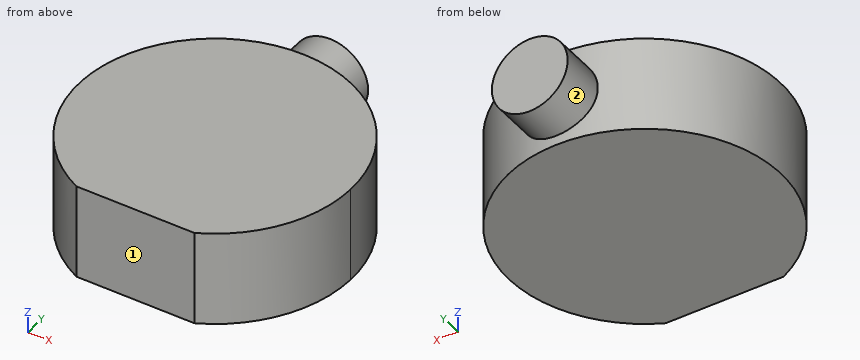
```python
from build123d import *

# Parameters (mm, degrees)
SKETCH_1_R          = 50
EXTRUDE_1_DEPTH     = 35
SKETCH_2_R          = 14
EXTRUDE_2_DEPTH     = 65
CUT_EXTRUDE_START   = -110
SKETCH_3_W          = 150
SKETCH_3_H          = 100
CUT_EXTRUDE_1_DEPTH = 64


with BuildPart() as part:
    # 草图1 → 凸台-拉伸1 (new body)
    with BuildSketch(Plane.XY):
        Circle(SKETCH_1_R)
    extrude(amount=EXTRUDE_1_DEPTH)

    # 草图2 → 凸台-拉伸2 (add)
    with BuildSketch(Plane(origin=(0, 0, 0), x_dir=(1, 0, 0), z_dir=(0, 1, 0))):
        with Locations((0, -17.5)):
            Circle(SKETCH_2_R)
    extrude(amount=EXTRUDE_2_DEPTH)

    # 草图3 → 切除-拉伸1 (cut)
    with BuildSketch(Plane(origin=(0, 65, 0), x_dir=(1, 0, 0), z_dir=(0, 1, 0)).offset(CUT_EXTRUDE_START)):
        Rectangle(SKETCH_3_W, SKETCH_3_H)
    extrude(amount=-CUT_EXTRUDE_1_DEPTH, mode=Mode.SUBTRACT)


solid = part.part
```
The listing builds one solid part. Answer for the finished solid, in the listing's coordinates (mm). Face numbers are marked on the shaded views. A direction names the side the tool comes from. Coordinates: 2 decimals unless noted, no trailing zeros. Write each loop counter-clockwise with the first axis right and the second up, starting at its lowest first coordinate (ties: lowest second). Pieces come first, ordered by that corner, then holes. Notation, with made-up numbers: (60.25, 33) - (110.25, 33) arc R26 ccw to (110.25, 70) - close; hole circle Ø10 at (-0.75, 67.5). An arc over 180 degrees is marked (long way). One line per item, written item: value.
1) A tool of negligible diameter and unlimited length cuts with its end or side. For the marked faces 1 and 2, from which of +Z, -Z, +X, -X, +Y, -Y can it reach the whole face along a straight path? Write none if from no direction.
Geometry check:
face 1: +Z, -Z, +X, -X, -Y
face 2: +Y
2) Find section D-D (z = 9.5). Give the vertices of the cut face in (x, y), and give its area (3 significant figures).
Geometry check:
outline: (-21.79, -45) - (21.79, -45) arc R50 ccw to (11.49, 48.66) - (11.49, 65) - (-11.49, 65) - (-11.49, 48.66) arc R50 ccw to start
area: 8,060 mm2
3) Find section B-B (z = 17.5). Give the vertices of the cut face in (x, y), and give its area (3 significant figures).
Geometry check:
outline: (-21.79, -45) - (21.79, -45) arc R50 ccw to (14, 48) - (14, 65) - (-14, 65) - (-14, 48) arc R50 ccw to start
area: 8,150 mm2
4) Find section C-C (y = 18). Give the vertices of the cut face in (x, z), and give its area (3 significant figures).
Geometry check:
outline: (-46.65, 0) - (46.65, 0) - (46.65, 35) - (-46.65, 35) - close
area: 3,270 mm2
5) Find section A-A (x = 0). Give the vertices of the cut face in (y, z).
Geometry check:
outline: (-45, 0) - (50, 0) - (50, 3.5) - (65, 3.5) - (65, 31.5) - (50, 31.5) - (50, 35) - (-45, 35) - close
6) Consider line 1 along X through (y, z) = (1, 6.5); line 2 along X through (y, z) = (14, 30.5); line 3 along Y through (x, z) = (-42, 18.5). Determine where each line is inside the solid, lowest interval first. Write a range as from..to.
Geometry check:
line 1: x = -49.99..49.99
line 2: x = -48..48
line 3: y = -27.13..27.13
7) Each of these flat-tipped pins is pushed along its axis until it touches: pin 1 Ø6 at (y, z) = (23.5, 5) entering from -X; pin 2 Ø3 at (x, z) = (-15.5, 9.5) entering from +Y; pin 3 Ø10 at (y, z) = (-30.5, 6) entering from -X. Where does it stop, or does it pass through?
Geometry check:
pin 1: stops at x = -45.6
pin 2: stops at y = 48
pin 3: stops at x = -43.01
